from build123d import *

# Parameters (mm, degrees)
BOSS_EXTRUDE1_OUTLINE_R   = 42
BOSS_EXTRUDE1_OUTLINE_R_2 = 2.1
BOSS_EXTRUDE1_OUTLINE_R_3 = 3.55
BOSS_EXTRUDE1_DEPTH       = 8
CUT_EXTRUDE2_DEPTH        = 10
BOSS_EXTRUDE5_DEPTH       = 10
SKETCH9_W                 = 3.6
SKETCH9_H                 = 3.6
BOSS_EXTRUDE6_DEPTH       = 8
FILLET1_R                 = 0.4


# Read off the part's stored shape, not the designer's step: Boss-Extrude1
with BuildPart() as part:
    # Boss-Extrude1 outline → Boss-Extrude1 (new body)
    with BuildSketch(Plane(origin=(0, 0, 0), x_dir=(1, 0, 0), z_dir=(0, 1, 0))):
        Circle(BOSS_EXTRUDE1_OUTLINE_R)
        with Locations((-15.588457268, -9)):
            Circle(BOSS_EXTRUDE1_OUTLINE_R_2, mode=Mode.SUBTRACT)
        with Locations((15.588457268, -9)):
            Circle(BOSS_EXTRUDE1_OUTLINE_R_2, mode=Mode.SUBTRACT)
        Circle(BOSS_EXTRUDE1_OUTLINE_R_3, mode=Mode.SUBTRACT)
        with Locations((0, 18)):
            Circle(BOSS_EXTRUDE1_OUTLINE_R_2, mode=Mode.SUBTRACT)
    extrude(amount=BOSS_EXTRUDE1_DEPTH)

    # Sketch3 → Cut-Extrude2 (cut)
    with BuildSketch(Plane(origin=(0, 8, 0), x_dir=(1, 0, 0), z_dir=(0, 1, 0))):
        with BuildLine():
            Line((0.5, 6), (0.5, 0))
            ThreePointArc((0.5, 0), (0, -0.5), (-0.5, 0))
            Line((-0.5, 0), (-0.5, 6))
            ThreePointArc((-0.5, 6), (0, 6.5), (0.5, 6))
        make_face()
    extrude(amount=-CUT_EXTRUDE2_DEPTH, mode=Mode.SUBTRACT)

    # Sketch7 → Boss-Extrude5 (add)
    with BuildSketch(Plane(origin=(0, 8, 0), x_dir=(1, 0, 0), z_dir=(0, 1, 0))):
        with BuildLine():
            Line((-5.196152423, -15), (0, -18))
            ThreePointArc((0, -18), (1.923015451, -16.253248712), (3.712435565, -14.369872981))
            Line((3.712435565, -14.369872981), (-2.696152423, -10.669872981))
            Line((-2.696152423, -10.669872981), (-5.196152423, -15))
        make_face()
        with BuildLine():
            Line((-10.392304845, 12), (-15.588457268, 9))
            ThreePointArc((-15.588457268, 9), (-15.037234004, 6.461244123), (-14.300892833, 3.969872981))
            Line((-14.300892833, 3.969872981), (-7.892304845, 7.669872981))
            Line((-7.892304845, 7.669872981), (-10.392304845, 12))
        make_face()
        with BuildLine():
            Line((15.588457268, 3), (15.588457268, 9))
            ThreePointArc((15.588457268, 9), (13.114218553, 9.792004588), (10.588457268, 10.4))
            Line((10.588457268, 10.4), (10.588457268, 3))
            Line((10.588457268, 3), (15.588457268, 3))
        make_face()
    extrude(amount=BOSS_EXTRUDE5_DEPTH)

    # Sketch9 → Boss-Extrude6 (add)
    with BuildSketch(Plane(origin=(0, 18, 0), x_dir=(1, 0, 0), z_dir=(0, 1, 0))):
        with Locations((13.688457268, 4.9)):
            Rectangle(SKETCH9_W, SKETCH9_H)
        Polygon((-0.141858429, -13.645706006), (-3.259549882, -11.845706006), (-5.059549882, -14.96339746), (-1.941858429, -16.76339746), align=None)
        Polygon((-11.746598839, 6.945706006), (-8.628907386, 8.745706006), (-10.428907386, 11.86339746), (-13.546598839, 10.06339746), align=None)
    extrude(amount=BOSS_EXTRUDE6_DEPTH)

    # Fillet1
    fillet1_edges = [part.edges().sort_by_distance(p)[0] for p in [
        (-13.546598839, 22, -10.06339746),
        (-11.746598839, 22, -6.945706006),
        (-8.628907386, 22, -8.745706006),
        (-10.428907386, 22, -11.86339746),
        (-7.892304845, 13, -7.669872981),
        (-10.392304845, 13, -12),
        (-15.588457268, 13, -9),
        (-14.300892833, 13, -3.969872981),
        (-2.696152423, 13, 10.669872981),
        (-5.196152423, 13, 15),
        (0, 13, 18),
        (3.712435565, 13, 14.369872981),
        (10.588457268, 13, -3),
        (15.588457268, 13, -3),
        (15.588457268, 13, -9),
        (10.588457268, 13, -10.4),
        (15.488457268, 22, -6.7),
        (11.888457268, 22, -6.7),
        (11.888457268, 22, -3.1),
        (15.488457268, 22, -3.1),
        (-1.941858429, 22, 16.76339746),
        (-0.141858429, 22, 13.645706006),
        (-3.259549882, 22, 11.845706006),
        (-5.059549882, 22, 14.96339746),
    ]]
    fillet(fillet1_edges, radius=FILLET1_R)


solid = part.part
Here's how the part is built. I have some questions about the finished solid (model axes, mm). A direction names the side the tool comes from. Round coordinates to 2 decimals unless told otherwise and drop trailing zeros. Order: outer loops, then holes, each group sorted by start corner. A loop starts at its lowest first (then second) coordinate and runs counter-clockwise, first axis right, second up. Notation, with made-up numbers: M 38.25,-11 L 44.25,-11 A17 ccw 44.25,-5 Z; hole C 25.5,49.25 d6. An arc over 180 degrees is marked long. Return JSON: item names as keys, results as strings. Group by question number.
1. I'm going to push flat-ended pins straight in: pin 1 Ø6 at (x, y) = (-16, 14) entering from -Z; pin 2 Ø0.8 at (y, z) = (23, -4.5) entering from -X; pin 3 Ø5 at (x, z) = (0, -18) entering from +Y. Where does each tip first touch, or does it pass through?
2. Please list where these lines run through material, in increasing order: probe 1 along Z at (x, y) = (0, 3.25); probe 2 along X at (y, z) = (2.75, 0); probe 3 along X at (y, z) = (4.75, 9).
3. If we mould it in two halves opening along X, with no side actions, what happens to faces 6 (the face through (13, 13, -3)), 7 (the face through (-9.52, 21.94, -10.29)), 8 (the face through (-11.1, 12.93, -5.82)), 9 (the face through (-0.149, 3.944, 3.547))? For each: pulls with the +X half, pulls with the -X half, needs draft (parallel to the pull), parting line crosses it, or undercut.
4. If we section it at C-C on y = 3.25: List the corners of the cut face in (x, z) for me, then the cut area to 3 significant figures.
5. On a 3-axis mill with a long thin cutter (end or side, diameter ignored), from which of +Z, -Z, +X, -X, +Y, -Y can I reach the whole of each face in a straight line? I mean faces 1 (the face through (-15.07, 12.93, -6.59)), 2 (the face through (0.51, 12.93, 12.52)), 3 (the face through (0.5, 4, -5)), 4 (the face through (1.825, 12.93, 16.349)), 5 (the face through (14, 22, -6.7)). Say none if no direction works.
6. If we section it at D-D on z = 9: List the corners of the cut face in (x, y) for me, then the cut area to 3 significant figures.
7. If we section it at B-B on z = 0: List the corners of the cut face in (x, y) for me, then the cut area to 3 significant figures.
8. If we section it at A-A on y = 15.5: List the corners of the cut face in (x, z) for me, then the cut area to 3 significant figures.
Reply:
{
 "1": {"pin 1": "z = -10.49", "pin 2": "x = 11.89", "pin 3": "y = 8"},
 "2": {"probe 1": "-42 to -20.1, -15.9 to -6.5, 3.55 to 42", "probe 2": "-42 to -3.55, 3.55 to 42", "probe 3": "-41.02 to -17.69, -13.49 to 13.49, 17.69 to 41.02"},
 "3": {"face 6": "needs draft", "face 7": "pulls with the +X half", "face 8": "undercut", "face 9": "undercut"},
 "4": {"outline": "C 0,0 d84; hole C -15.59,9 d4.2; hole C 0,-18 d4.2; hole M -0.5,-6 A0.5 ccw 0.5,-6 L 0.5,-3.51 A3.55 ccw long -0.5,-3.51 Z; hole C 15.59,9 d4.2", "area": "5,460 mm^2"},
 "5": {"face 1": "+Z, -X, +Y", "face 2": "-Z, +X, +Y", "face 3": "+Y, -Y", "face 4": "+Z, +X, +Y", "face 5": "-Z, +X, -X, +Y"},
 "6": {"outline": "M -41.02,0 L -17.69,0 L -17.69,8 L -41.02,8 Z; M -13.49,0 L 13.49,0 L 13.49,8 L -13.49,8 Z; M 17.69,0 L 41.02,0 L 41.02,8 L 17.69,8 Z", "area": "589 mm^2"},
 "7": {"outline": "M -42,0 L -3.55,0 L -3.55,8 L -42,8 Z; M 3.55,0 L 42,0 L 42,8 L 3.55,8 Z", "area": "615 mm^2"},
 "8": {"outline": "M -15.54,-8.72 A0.4 ccw -15.34,-9.14 L -10.74,-11.8 A0.4 ccw -10.19,-11.65 L -8.09,-8.02 A0.4 ccw -8.24,-7.47 L -13.87,-4.22 A0.4 ccw -14.46,-4.44 A35.32 ccw Z; M -5,14.65 L -2.9,11.02 A0.4 ccw -2.35,10.87 L 3.29,14.12 A0.4 ccw 3.38,14.74 A35.32 ccw 0.22,17.82 A0.4 ccw -0.24,17.86 L -4.85,15.2 A0.4 ccw Z; M 10.59,-9.91 A0.4 ccw 11.07,-10.3 A35.32 ccw 15.32,-9.1 A0.4 ccw 15.59,-8.72 L 15.59,-3.4 A0.4 ccw 15.19,-3 L 10.99,-3 A0.4 ccw 10.59,-3.4 Z", "area": "101 mm^2"}
}
